The listing builds one solid part. Answer for the finished solid, in the listing's coordinates (mm). Face numbers are marked on the shaded views. A direction names the side the tool comes from. Round coordinates to 2 decimals unless told otherwise and drop trailing zeros. Order: outer loops, then holes, each group sorted by start corner. A loop starts at its lowest first (then second) coordinate and runs counter-clockwise, first axis right, second up. Notation, with made-up numbers: M 21.25,-6 L 52.25,-6 A11 ccw 52.25,7 Z; hole C -34.5,8 d9. An arc over 180 degrees is marked long. Put each result on its own line as item: value. Start each with the question number.
1. Consider line 1 (X direction, y = 64, z = 15.75); line 2 (Y direction, x = 6, z = 19.25); line 3 (X direction, y = 7, z = 9.5). Determine where each line is inside the solid, lowest interval first.
2. The part is cut by section C-C (x = 9). Give the vertices of the cut face in (y, z).
3. Each of these flat-tipped pins is pushed along its axis until it touches: pin 1 Ø6 at (x, z) = (38.5, 11.5) entering from -Y; pin 2 Ø10 at (y, z) = (33.5, 17.5) entering from +X; pin 3 Ø1.4 at (y, z) = (2.5, 7.5) entering from -X; pin 4 Ø4 at (x, y) = (25, 29.5) entering from +Z. Where does it stop, or does it pass through?
4. The mould has two halves that part along Y. Classify the marked faces 1, 2 and 3: +Y half, -Y half, draft (parallel to the pull), parting line (faces both ways), or undercut.
5. The part is cut by section D-D (x = 38.5). Give the vertices of the cut face in (y, z).
6. The part is cut by section A-A (x = 20). Give the vertices of the cut face in (y, z).
7. The part is cut by section B-B (y = 31). Give the vertices of the cut face in (x, z), then the cut area to 3 significant figures.
8. Which of the six approach directions +Z, -Z, +X, -X, +Y, -Y give full straight-line access (tool end or side, diameter ignored) to the marked faces 4, 5 and 6?
from build123d import *

# Parameters (mm, degrees)
SKETCH1_W                        = 75
SKETCH1_H                        = 70
BASE_FLANGE1_DEPTH               = 1.29
EDGE_FLANGE1_STRIP_W             = 6.684
EDGE_FLANGE1_STRIP_H             = 1.29
EDGE_FLANGE1_STRIP_CUT_DEPTH     = 75
EDGE_FLANGE1_DEPTH               = 75
EDGE_FLANGE2_STRIP_W             = 6.684
EDGE_FLANGE2_STRIP_H             = 1.29
EDGE_FLANGE2_STRIP_CUT_DEPTH     = 75
EDGE_FLANGE2_DEPTH               = 75
EDGE_FLANGE3_STRIP_W             = 6.684
EDGE_FLANGE3_STRIP_H             = 1.29
EDGE_FLANGE3_STRIP_CUT_DEPTH     = 65.896
EDGE_FLANGE3_DEPTH               = 65.896
EDGE_FLANGE4_STRIP_W             = 6.684
EDGE_FLANGE4_STRIP_H             = 1.29
EDGE_FLANGE4_STRIP_CUT_DEPTH     = 65.896
EDGE_FLANGE4_DEPTH               = 65.896
EDGE_FLANGE6_START               = 1.117
EDGE_FLANGE6_DEPTH               = 18.883
EDGE_FLANGE6_2_DEPTH             = 0.645
EDGE_FLANGE6_START_2             = 1.762
EDGE_FLANGE6_3_DEPTH             = 18.238
EDGE_FLANGE8_START               = 1.117
EDGE_FLANGE8_DEPTH               = 18.883
EDGE_FLANGE8_2_DEPTH             = 0.645
EDGE_FLANGE8_START_2             = 1.762
EDGE_FLANGE8_3_DEPTH             = 18.238
EDGE_FLANGE9_DEPTH               = 19.238
EDGE_FLANGE10_DEPTH              = 19.238
TAP_DRILL_FOR_M4X0_7_TAP1_REACH  = 108.005
TAP_DRILL_FOR_M4X0_7_TAP1_BORE_R = 1.65
M3_CLEARANCE_HOLE1_D             = 3.4
M3_CLEARANCE_HOLE1_DEPTH         = 3.342
M3_CLEARANCE_HOLE2_D             = 3.4


# Read off the part's stored shape, not the designer's step: Edge-Flange6, Edge-Flange8
# Sheet-metal steps are written as plain solids
with BuildPart() as part:
    # Sketch1 → Base-Flange1 (new body)
    with BuildSketch(Plane.XY):
        with Locations((37.5, 35)):
            Rectangle(SKETCH1_W, SKETCH1_H)
    extrude(amount=-BASE_FLANGE1_DEPTH)

    # Edge-Flange1 strip (across the edge) → Edge-Flange1 strip cut (cut)
    with BuildSketch(Plane(origin=(75, 70, 0), x_dir=(0, -1, 0), z_dir=(-1, 0, 0))):
        with Locations((-1.29, -0.645)):
            Rectangle(EDGE_FLANGE1_STRIP_W, EDGE_FLANGE1_STRIP_H)
    extrude(amount=EDGE_FLANGE1_STRIP_CUT_DEPTH, mode=Mode.SUBTRACT)

    # Edge-Flange1 section (across the edge) → Edge-Flange1 (add)
    with BuildSketch(Plane(origin=(75, 70, 0), x_dir=(0, -1, 0), z_dir=(-1, 0, 0))):
        with BuildLine():
            Line((0, 0.762), (0, 20))
            Line((0, 20), (1.29, 20))
            Line((1.29, 20), (1.29, 0.762))
            ThreePointArc((1.29, 0.762), (1.513184633, 0.223184633), (2.052, 0))
            Line((2.052, 0), (2.052, -1.29))
            ThreePointArc((2.052, -1.29), (0.601016885, -0.688983115), (0, 0.762))
        make_face()
    extrude(amount=EDGE_FLANGE1_DEPTH)

    # Edge-Flange2 strip (across the edge) → Edge-Flange2 strip cut (cut)
    with BuildSketch(Plane.YZ):
        with Locations((-1.29, -0.645)):
            Rectangle(EDGE_FLANGE2_STRIP_W, EDGE_FLANGE2_STRIP_H)
    extrude(amount=EDGE_FLANGE2_STRIP_CUT_DEPTH, mode=Mode.SUBTRACT)

    # Edge-Flange2 section (across the edge) → Edge-Flange2 (add)
    with BuildSketch(Plane.YZ):
        with BuildLine():
            Line((0, 0.762), (0, 20))
            Line((0, 20), (1.29, 20))
            Line((1.29, 20), (1.29, 0.762))
            ThreePointArc((1.29, 0.762), (1.513184633, 0.223184633), (2.052, 0))
            Line((2.052, 0), (2.052, -1.29))
            ThreePointArc((2.052, -1.29), (0.601016885, -0.688983115), (0, 0.762))
        make_face()
    extrude(amount=EDGE_FLANGE2_DEPTH)

    # Edge-Flange3 strip (across the edge) → Edge-Flange3 strip cut (cut)
    with BuildSketch(Plane.XZ.offset(-67.948)):
        with Locations((-1.29, -0.645)):
            Rectangle(EDGE_FLANGE3_STRIP_W, EDGE_FLANGE3_STRIP_H)
    extrude(amount=EDGE_FLANGE3_STRIP_CUT_DEPTH, mode=Mode.SUBTRACT)

    # Edge-Flange3 section (across the edge) → Edge-Flange3 (add)
    with BuildSketch(Plane.XZ.offset(-67.948)):
        with BuildLine():
            Line((0, 0.762), (0, 20))
            Line((0, 20), (1.29, 20))
            Line((1.29, 20), (1.29, 0.762))
            ThreePointArc((1.29, 0.762), (1.513184633, 0.223184633), (2.052, 0))
            Line((2.052, 0), (2.052, -1.29))
            ThreePointArc((2.052, -1.29), (0.601016885, -0.688983115), (0, 0.762))
        make_face()
    extrude(amount=EDGE_FLANGE3_DEPTH)

    # Edge-Flange4 strip (across the edge) → Edge-Flange4 strip cut (cut)
    with BuildSketch(Plane(origin=(75, 2.052, 0), x_dir=(-1, 0, 0), z_dir=(0, 1, 0))):
        with Locations((-1.29, -0.645)):
            Rectangle(EDGE_FLANGE4_STRIP_W, EDGE_FLANGE4_STRIP_H)
    extrude(amount=EDGE_FLANGE4_STRIP_CUT_DEPTH, mode=Mode.SUBTRACT)

    # Edge-Flange4 section (across the edge) → Edge-Flange4 (add)
    with BuildSketch(Plane(origin=(75, 2.052, 0), x_dir=(-1, 0, 0), z_dir=(0, 1, 0))):
        with BuildLine():
            Line((0, 0.762), (0, 20))
            Line((0, 20), (1.29, 20))
            Line((1.29, 20), (1.29, 0.762))
            ThreePointArc((1.29, 0.762), (1.513184633, 0.223184633), (2.052, 0))
            Line((2.052, 0), (2.052, -1.29))
            ThreePointArc((2.052, -1.29), (0.601016885, -0.688983115), (0, 0.762))
        make_face()
    extrude(amount=EDGE_FLANGE4_DEPTH)

    # Edge-Flange6 outline → Edge-Flange6 (cut)
    with BuildSketch(Plane.XY.offset(EDGE_FLANGE6_START)):
        with BuildLine():
            Line((1.29, 2.052), (1.29, 2.198728366))
            ThreePointArc((1.29, 2.198728366), (0.352834322, 2.953547915), (0, 4.104))
            Line((0, 4.104), (0, 2.052))
            Line((0, 2.052), (1.29, 2.052))
        make_face()
    extrude(amount=EDGE_FLANGE6_DEPTH, mode=Mode.SUBTRACT)

    # Edge-Flange6 2 outline → Edge-Flange6 2 (cut)
    with BuildSketch(Plane.XY.offset(EDGE_FLANGE6_START)):
        with BuildLine():
            ThreePointArc((0, 4.104), (0.352834322, 2.953547915), (1.29, 2.198728366))
            Line((1.29, 2.198728366), (1.29, 4.749))
            Line((1.29, 4.749), (0, 4.749))
            Line((0, 4.749), (0, 4.104))
        make_face()
    extrude(amount=EDGE_FLANGE6_2_DEPTH, mode=Mode.SUBTRACT)

    # Edge-Flange6 3 outline → Edge-Flange6 3 (add)
    with BuildSketch(Plane.XY.offset(EDGE_FLANGE6_START_2)):
        with BuildLine():
            Line((2.052, 2.052), (16.29, 2.052))
            Line((16.29, 2.052), (16.29, 3.342))
            Line((16.29, 3.342), (2.052, 3.342))
            ThreePointArc((2.052, 3.342), (1.513184633, 3.565184633), (1.29, 4.104))
            Line((1.29, 4.104), (1.29, 2.198728366))
            ThreePointArc((1.29, 2.198728366), (1.664000898, 2.089015956), (2.052, 2.052))
        make_face()
    extrude(amount=EDGE_FLANGE6_3_DEPTH)

    # Edge-Flange8 outline → Edge-Flange8 (cut)
    with BuildSketch(Plane.XY.offset(EDGE_FLANGE8_START)):
        with BuildLine():
            ThreePointArc((75, 4.104), (74.647165678, 2.953547915), (73.71, 2.198728366))
            Line((73.71, 2.198728366), (73.71, 2.052))
            Line((73.71, 2.052), (75, 2.052))
            Line((75, 2.052), (75, 4.104))
        make_face()
    extrude(amount=EDGE_FLANGE8_DEPTH, mode=Mode.SUBTRACT)

    # Edge-Flange8 2 outline → Edge-Flange8 2 (cut)
    with BuildSketch(Plane.XY.offset(EDGE_FLANGE8_START)):
        with BuildLine():
            Line((73.71, 4.749), (73.71, 2.198728366))
            ThreePointArc((73.71, 2.198728366), (74.647165678, 2.953547915), (75, 4.104))
            Line((75, 4.104), (75, 4.749))
            Line((75, 4.749), (73.71, 4.749))
        make_face()
    extrude(amount=EDGE_FLANGE8_2_DEPTH, mode=Mode.SUBTRACT)

    # Edge-Flange8 3 outline → Edge-Flange8 3 (add)
    with BuildSketch(Plane.XY.offset(EDGE_FLANGE8_START_2)):
        with BuildLine():
            Line((58.71, 2.052), (72.948, 2.052))
            ThreePointArc((72.948, 2.052), (73.335999102, 2.089015956), (73.71, 2.198728366))
            Line((73.71, 2.198728366), (73.71, 4.104))
            ThreePointArc((73.71, 4.104), (73.486815367, 3.565184633), (72.948, 3.342))
            Line((72.948, 3.342), (58.71, 3.342))
            Line((58.71, 3.342), (58.71, 2.052))
        make_face()
    extrude(amount=EDGE_FLANGE8_3_DEPTH)

    # Edge-Flange9 section (across the edge) → Edge-Flange9 (add)
    with BuildSketch(Plane(origin=(75.762, 68.71, 0.762), x_dir=(-1, 0, 0), z_dir=(0, 0, 1))):
        with BuildLine():
            Line((-1.29, 0.762), (-1.29, 15))
            Line((-1.29, 15), (0, 15))
            Line((0, 15), (0, 0.762))
            ThreePointArc((0, 0.762), (0.223184633, 0.223184633), (0.762, 0))
            Line((0.762, 0), (0.762, -1.29))
            ThreePointArc((0.762, -1.29), (-0.688983115, -0.688983115), (-1.29, 0.762))
        make_face()
    extrude(amount=EDGE_FLANGE9_DEPTH)

    # Edge-Flange10 section (across the edge) → Edge-Flange10 (add)
    with BuildSketch(Plane(origin=(-0.762, 68.71, 20), x_dir=(1, 0, 0), z_dir=(0, 0, -1))):
        with BuildLine():
            Line((-1.29, 0.762), (-1.29, 15))
            Line((-1.29, 15), (0, 15))
            Line((0, 15), (0, 0.762))
            ThreePointArc((0, 0.762), (0.223184633, 0.223184633), (0.762, 0))
            Line((0.762, 0), (0.762, -1.29))
            ThreePointArc((0.762, -1.29), (-0.688983115, -0.688983115), (-1.29, 0.762))
        make_face()
    extrude(amount=EDGE_FLANGE10_DEPTH)

    # Tap Drill for M4x0.7 Tap1 bore → Tap Drill for M4x0.7 Tap1 (cut, up to next)
    with BuildSketch(Plane(origin=(0, 70, 0), x_dir=(1, 0, 0), z_dir=(0, 1, 0)), mode=Mode.PRIVATE) as tap_drill_for_m4x0_7_tap1_sk1:
        with Locations((55, -10.381)):
            Circle(TAP_DRILL_FOR_M4X0_7_TAP1_BORE_R)
    tap_drill_for_m4x0_7_tap1_tool1 = extrude(tap_drill_for_m4x0_7_tap1_sk1.sketch, amount=-TAP_DRILL_FOR_M4X0_7_TAP1_REACH, mode=Mode.PRIVATE) & part.part
    # Tap Drill for M4x0.7 Tap1 bore → Tap Drill for M4x0.7 Tap1 (cut, up to next)
    with BuildSketch(Plane(origin=(0, 70, 0), x_dir=(1, 0, 0), z_dir=(0, 1, 0)), mode=Mode.PRIVATE) as tap_drill_for_m4x0_7_tap1_sk2:
        with Locations((20, -10.381)):
            Circle(TAP_DRILL_FOR_M4X0_7_TAP1_BORE_R)
    tap_drill_for_m4x0_7_tap1_tool2 = extrude(tap_drill_for_m4x0_7_tap1_sk2.sketch, amount=-TAP_DRILL_FOR_M4X0_7_TAP1_REACH, mode=Mode.PRIVATE) & part.part
    add(tap_drill_for_m4x0_7_tap1_tool1.solids().sort_by_distance((55, 70, 10.381))[0], mode=Mode.SUBTRACT)
    add(tap_drill_for_m4x0_7_tap1_tool2.solids().sort_by_distance((20, 70, 10.381))[0], mode=Mode.SUBTRACT)

    # M3 Clearance Hole1
    with Locations(Plane(origin=(0, 3.342, 0), x_dir=(1, 0, 0), z_dir=(0, 1, 0))):
        with Locations((9.171, -10.881), (65.829, -10.881)):
            Hole(M3_CLEARANCE_HOLE1_D / 2, depth=M3_CLEARANCE_HOLE1_DEPTH)

    # M3 Clearance Hole2 (through all)
    with Locations(Plane(origin=(77.052, 0, 0), x_dir=(0, 0, -1), z_dir=(1, 0, 0))):
        with Locations((-10.381, 60.829)):
            Hole(M3_CLEARANCE_HOLE2_D / 2)


solid = part.part
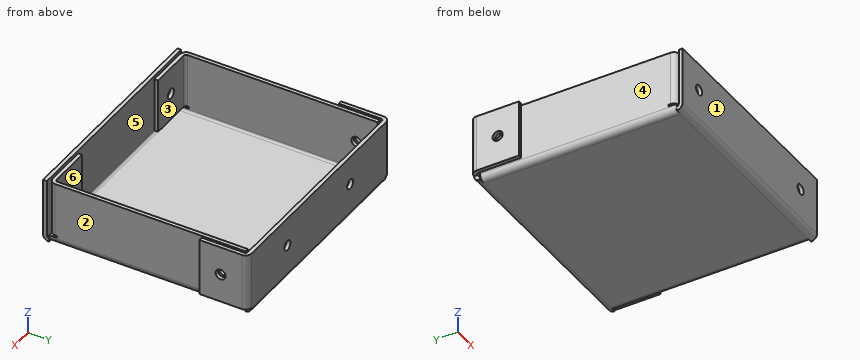
Resolved:
1. line 1: -2.05 to -0.76, 0 to 1.29, 73.71 to 75, 75.76 to 77.05
1. line 2: 0 to 1.29, 2.05 to 3.34, 68.71 to 70
1. line 3: 0 to 1.29, 73.71 to 75
2. outline: M 0,0.76 A2.05 ccw 2.05,-1.29 L 67.95,-1.29 A2.05 ccw 70,0.76 L 70,20 L 68.71,20 L 68.71,0.76 A0.76 cw 67.95,0 L 2.05,0 A0.76 cw 1.29,0.76 L 1.29,9.19 L 0,9.19 Z; M 0,12.57 L 1.29,12.57 L 1.29,20 L 0,20 Z; M 2.05,1.76 L 3.34,1.76 L 3.34,9.19 L 2.05,9.19 Z; M 2.05,12.57 L 3.34,12.57 L 3.34,20 L 2.05,20 Z
3. pin 1: y = 0
3. pin 2: x = 75
3. pin 3: x = 0.21
3. pin 4: z = 0
4. face 1: -Y half
4. face 2: draft
4. face 3: undercut
5. outline: M 0,0.76 A2.05 ccw 2.05,-1.29 L 67.95,-1.29 A2.05 ccw 70,0.76 L 70,20 L 68.71,20 L 68.71,0.76 A0.76 cw 67.95,0 L 2.05,0 A0.76 cw 1.29,0.76 L 1.29,20 L 0,20 Z
6. outline: M 0,0.76 A2.05 ccw 2.05,-1.29 L 67.95,-1.29 A2.05 ccw 70,0.76 L 70,8.73 L 68.71,8.73 L 68.71,0.76 A0.76 cw 67.95,0 L 2.05,0 A0.76 cw 1.29,0.76 L 1.29,20 L 0,20 Z; M 68.71,12.03 L 70,12.03 L 70,20 L 68.71,20 Z
7. outline: M 0,0.76 A2.05 ccw 2.05,-1.29 L 72.95,-1.29 A2.05 ccw 75,0.76 L 75,20 L 73.71,20 L 73.71,0.76 A0.76 cw 72.95,0 L 2.05,0 A0.76 cw 1.29,0.76 L 1.29,20 L 0,20 Z
7. area: 147 mm2
8. face 4: +Z, -Z, -Y
8. face 5: +Z, +X, -X
8. face 6: +Z
